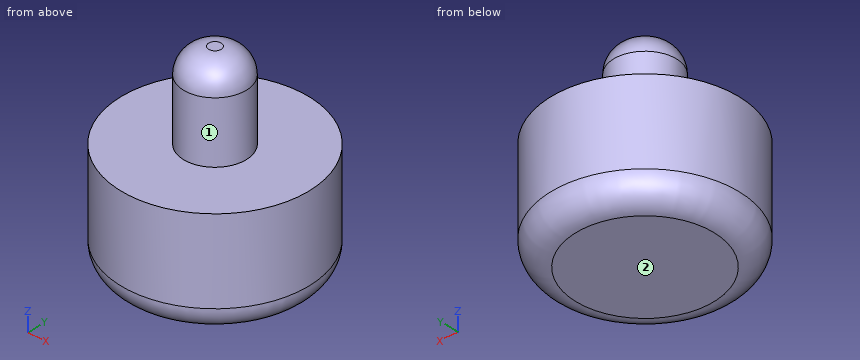
```python
from build123d import *

# Parameters (mm, degrees)
F0_R     = 9.525
F1_DEPTH = 11.049
F2_R     = 2.54
F3_R     = 3.175
F4_DEPTH = 8.763
F5_R     = 2.54


# Not quite as in the source:
# - a feature names something its author has since deleted; it is built from what else it names


with BuildPart() as f1:
    # F0 (on Top) → F1 (new body)
    with BuildSketch(Plane.XY):
        with Locations((-0.0108847216, 0.0162923955)):
            Circle(F0_R)
    extrude(amount=F1_DEPTH)

    # F2
    f2_edges = [f1.edges().sort_by_distance(p)[0] for p in [
        (-9.535885, 0.016292, 0),
    ]]
    fillet(f2_edges, radius=F2_R)

    # F3 (on face) → F4 (join)
    with BuildSketch(Plane.XY.offset(11.049)):
        Circle(F3_R)
    extrude(amount=F4_DEPTH)

    # F5
    f5_edges = [f1.edges().sort_by_distance(p)[0] for p in [
        (-3.175, 0, 19.812),
    ]]
    fillet(f5_edges, radius=F5_R)


solid = f1.part
```
Source: CAD feature listing. Evaluate the final solid. Frame: model axes, mm. Face numbers are marked on the shaded views. A direction names the side the tool comes from. Give positions to 0.01 mm unless a question says otherwise; leave off trailing zeros. Loops run counter-clockwise (first coordinate to the right, second up) from the corner with the lowest first, then second, coordinate; pieces in that order, holes last. Notation, with made-up numbers: (-19, -15.75) - (35, -15.75) arc R17 ccw to (35, -9.75) - close; hole circle Ø2 at (86, 63). An arc over 180 degrees is marked (long way). Use CSV: the item, a comma, the result in double quotes. Start each with the question number.
1. Pin query (flat end, axial travel): pin 1 (10 mm diameter, centred on x = 2.5, z = 16.5, fed in from -Y) (3 decimals); pin 2 (5 mm diameter, centred on y = 1, z = 15.5, fed in from -X) (3 decimals); pin 3 (1 mm diameter, centred on x = 5.5, y = -5.5, fed in from +Z). Return the tip coordinate at first contact, or that it passes through.
2. Section A-A (z = 12). Output: boundary loops of the cut face in (x, y) (3 decimals), then the cut area to 3 significant figures.
3. Section B-B (z = 7.5). Output: boundary loops of the cut face in (x, y) (3 decimals).
4. Reachability of the marked faces 1 and 2 from +Z, -Z, +X, -X, +Y, -Y: full face, straight path, thin tool, end or side. Return the list, or none.
5. Ray query, L1, parallel to Z at x = -4.75, y = 0; L2, parallel to X at y = -8.5, z = 3.75; L3, parallel to X at y = 1, z = 16. Return the intervals inside material, ascending.
Response:
1,pin 1,"y = -3.175"
1,pin 2,"x = -3.175"
1,pin 3,"z = 11.05"
2,outline,"circle Ø6.35 at (0, 0)"
2,area,"31.7 mm²"
3,outline,"circle Ø19.05 at (-0.011, 0.016)"
4,face 1,"+Z"
4,face 2,"-Z, +X, -X, +Y, -Y"
5,L1,"0 to 11.05"
5,L2,"-4.28 to 4.26"
5,L3,"-3.01 to 3.01"
